Autodesk Inventor part; units mm, degrees
ref_plane "YZ Plane" through (0, 0, 0) normal (1, 0, 0) x (0, 1, 0)
ref_plane "XZ Plane" through (0, 0, 0) normal (0, 1, 0) x (-1, 0, 0)
ref_plane "XY Plane" through (0, 0, 0) normal (0, 0, 1) x (1, 0, 0)
sketch "Esquisse1" plane through (0, 0, 0) normal (0, 1, 0) x (-1, 0, 0)
  line L0 (0, 0) -> (27, 0)
  line L1 (27, 0) -> (27, 27.55)
  line L2 (27, 27.55) -> (0, 27.55)
  line L3 (0, 27.55) -> (0, 0)
  circle A0 centre (4.65, 3.65) radius 2.15
  line L4 (13.5, 27.55) -> (13.5, 0) construction
  circle A1 centre (22.35, 3.65) radius 2.15
  dimension "d0" = 27
  dimension "d1" = 27.55
  dimension "d2" = 4.3
  dimension "d3" = 3.65
  dimension "d4" = 4.65
extrude "Extrusion1" add sketch "Esquisse1" along normal blind 2.2
sketch "Esquisse2" plane through (0, 0, 0) normal (0, -1, 0) x (1, 0, 0)
  line L0 (0, 27.55) -> (0, 0) construction
  line L1 (-27, 27.55) -> (0, 27.55)
  line L2 (0, 27.55) -> (0, 25.35)
  line L3 (0, 25.35) -> (-27, 25.35)
  line L4 (-27, 25.35) -> (-27, 27.55)
  dimension "d7" = 2.2
extrude "Extrusion2" add sketch "Esquisse2" along normal blind 5
sketch "Esquisse3" plane through (-27, 2.2, 27.55) normal (0, 0, 1) x (1, 0, 0)
  line L0 (27, -7.2) -> (27, 0) construction
  line L1 (0, -7.2) -> (0, 0) construction
  line L2 (27, -7.2) -> (0, -7.2) construction
  line L3 (0, -4.2) -> (27, -4.2) construction
  circle A0 centre (13.5, -4.2) radius 1.3
  circle A1 centre (18.5, -4.2) radius 1.3
  circle A2 centre (8.5, -4.2) radius 1.3
  circle A3 centre (13.5, -4.2) radius 1.3
  point P0 (27, -2.2)
  dimension "d10" = 3
  dimension "d11" = 2.6
  dimension "d14" = 5
  dimension "d17" = 5
extrude "Extrusion3" cut sketch "Esquisse3" against normal through all
properties part number "BodyToOpenCM"
Part model, mm, in its own coordinate system. A direction names the side the tool comes from. Coordinates: 2 decimals unless noted, no trailing zeros. Order: outer loops, then holes, each group sorted by start corner. A loop starts at its lowest first (then second) coordinate and runs counter-clockwise, first axis right, second up.
(1) Slice it at C-C, the plane x = -22.35. Write the cut outline in (y, z).
Check sheet entries:
outline: (-5, 25.35) - (0, 25.35) - (0, 5.8) - (2.2, 5.8) - (2.2, 27.55) - (-5, 27.55) - close; (0, 0) - (2.2, 0) - (2.2, 1.5) - (0, 1.5) - close
(2) Slice it at A-A, the plane x = -8.5. Write the cut outline in (y, z), and give its area (3 significant figures).
Check sheet entries:
outline: (-5, 25.35) - (-3.3, 25.35) - (-3.3, 27.55) - (-5, 27.55) - close; (-0.7, 25.35) - (0, 25.35) - (0, 0) - (2.2, 0) - (2.2, 27.55) - (-0.7, 27.55) - close
area: 65.9 mm2
(3) Slice it at D-D, the plane z = 23.5. Write the cut outline in (x, y).
Check sheet entries:
outline: (-27, 0) - (0, 0) - (0, 2.2) - (-27, 2.2) - close
(4) Pin check, flat tips, straight feed: pin 1 Ø7 at (x, z) = (-4.65, 3.65) entering from -Y; pin 2 Ø3.5 at (x, y) = (-13.5, -2) entering from -Z. Stop position of each tip, or through.
Check sheet entries:
pin 1: stops at y = 0
pin 2: stops at z = 25.35
(5) Slice it at B-B, the plane y = -2. Write the cut outline in (x, z), and give its area (3 significant figures).
Check sheet entries:
outline: (-27, 25.35) - (-19.8, 25.35) - (-19.8, 27.55) - (-27, 27.55) - close; (-17.2, 25.35) - (-14.8, 25.35) - (-14.8, 27.55) - (-17.2, 27.55) - close; (-12.2, 25.35) - (-9.8, 25.35) - (-9.8, 27.55) - (-12.2, 27.55) - close; (-7.2, 25.35) - (0, 25.35) - (0, 27.55) - (-7.2, 27.55) - close
area: 42.2 mm2
(6) Probe L1, parallel to Y at x = -8.5, z = 26.2; L2, parallel to Z at x = -22.35, y = 1.6; L3, parallel to Z at x = -16, y = -0.5. List the from-to ranges inside material, lowest first.
Check sheet entries:
L1: y = -5 to -3.3, -0.7 to 2.2
L2: z = 0 to 1.5, 5.8 to 27.55
L3: z = 25.35 to 27.55
(7) Pull direction Y, two halves, no side cores. Call faces 1 (the face through (-24.4, 1.1, 3)), 2 (the face through (-14.53, -2.79, 26.47)), 3 (the face through (-13, 2.2, 14)): pulls with the +Y half, pulls with the -Y half, needs draft (parallel to the pull), parting line crosses it, or undercut.
Check sheet entries:
face 1: needs draft
face 2: undercut
face 3: pulls with the +Y half
(8) Tool access for faces 4 (the face through (-13, -4, 25.35)), 5 (the face through (-19.8, -1.94, 26.47)): list every direction of +Z, -Z, +X, -X, +Y, -Y with a clear straight run to the whole face (end or side of a thin tool).
Check sheet entries:
face 4: -Z, +X, -X, -Y
face 5: +Z, -Z
